Design review of the part built by this model. Coordinates are the model's own, in mm. Face numbers are marked on the shaded views. Give positions to 0.01 mm unless a question says otherwise; leave off trailing zeros. Order: outer loops, then holes, each group sorted by start corner. A loop starts at its lowest first (then second) coordinate and runs counter-clockwise, first axis right, second up. Notation, with made-up numbers: M 10,-12.75 L 52,-12.75 A31 ccw 52,26.25 Z; hole C -1,-14 d1. An arc over 180 degrees is marked long. Put each result on its own line as item: value. Start each with the question number.
from build123d import *

# Parameters (mm, degrees)
SKETCH5_W              = 55.1
SKETCH5_H              = 15
BASE_FLANGE1_DEPTH     = 0.6
SKETCHED_START         = -27.55
SKETCHED_BEND2_DEPTH   = 55.1
SKETCHED_BEND2_2_DEPTH = 55.1


# Read off the part's stored shape, not the designer's step: Sketched Bend2
# Sheet-metal steps are written as plain solids
with BuildPart() as part:
    # Sketch5 → Base-Flange1 (new body)
    with BuildSketch(Plane(origin=(0, 0, 0), x_dir=(1, 0, 0), z_dir=(0, 1, 0))):
        Rectangle(SKETCH5_W, SKETCH5_H)
    extrude(amount=-BASE_FLANGE1_DEPTH)

    # Sketched Bend2 outline → Sketched Bend2 (cut)
    with BuildSketch(Plane.YZ.offset(SKETCHED_START)):
        with BuildLine():
            ThreePointArc((-0.6, -1.247910415), (-0.44222051, -0.555090092), (0, 0.001089185))
            Line((0, 0.001089185), (0, 7.5))
            Line((0, 7.5), (-0.6, 7.5))
            Line((-0.6, 7.5), (-0.6, -1.247910415))
        make_face()
    extrude(amount=SKETCHED_BEND2_DEPTH, mode=Mode.SUBTRACT)

    # Sketched Bend2 2 outline → Sketched Bend2 2 (add)
    with BuildSketch(Plane.YZ.offset(SKETCHED_START)):
        with BuildLine():
            Line((7.217062591, -2.44655837), (7.422274677, -1.882742798))
            Line((7.422274677, -1.882742798), (1.547232229, 0.255597778))
            ThreePointArc((1.547232229, 0.255597778), (0.740301483, 0.330872876), (0, 0.001089185))
            Line((0, 0.001089185), (0, -1.247910415))
            ThreePointArc((0, -1.247910415), (0.426423564, -0.428758371), (1.342020143, -0.308217794))
            Line((1.342020143, -0.308217794), (7.217062591, -2.44655837))
        make_face()
    extrude(amount=SKETCHED_BEND2_2_DEPTH)


solid = part.part
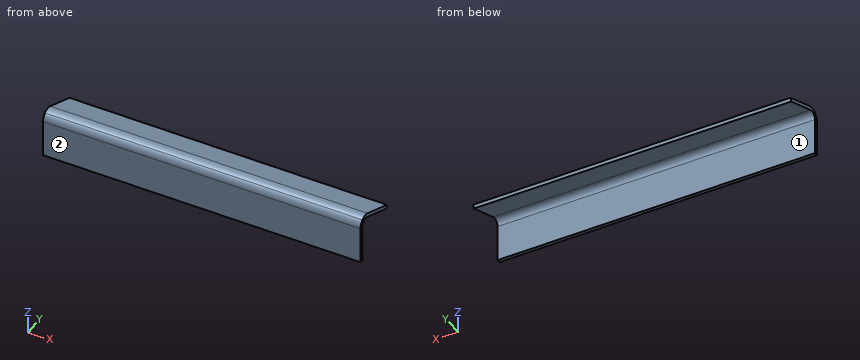
1. The part is to be moulded in two halves that separate along Y. For the marked faces 1 and 2, say which applies: +Y half, -Y half, draft (parallel to the pull), parting line (faces both ways), or undercut.
2. To check wall thickness, follow probe 1 along Z at (x, y) = (-20, 1); probe 2 along Y at (x, z) = (9, -6); probe 3 along Z at (x, y) = (18, 5). State the ranges of each line that lie inside material, in increasing order.
3. Consider section B-B on z = -6.25. Give the boundary of the cut face in (x, y), then the cut area to 3 significant figures.
4. Consider section A-A on x = 12. Give the boundary of the cut face in (y, z), then the cut area to 3 significant figures.
5. Consider section C-C on y = 6.5. Give the boundary of the cut face in (x, z).
Returned:
1. face 1: undercut
1. face 2: -Y half
2. probe 1: z = -0.25 to 0.35
2. probe 2: y = -0.6 to 0
2. probe 3: z = -1.64 to -1
3. outline: M -27.55,-0.6 L 27.55,-0.6 L 27.55,0 L -27.55,0 Z
3. area: 33.1 mm2
4. outline: M -0.6,-7.5 L 0,-7.5 L 0,-1.25 A1 cw 1.34,-0.31 L 7.22,-2.45 L 7.42,-1.88 L 1.55,0.26 A1.6 ccw -0.6,-1.25 Z
4. area: 9.00 mm2
5. outline: M -27.55,-2.19 L 27.55,-2.19 L 27.55,-1.55 L -27.55,-1.55 Z
